from build123d import *

# Parameters (mm, degrees)
SKETCH1_W           = 57
SKETCH1_H           = 24.4
BOSS_EXTRUDE1_DEPTH = 1.2
SKETCH2_R           = 1.5
CUT_EXTRUDE1_DEPTH  = 2.2
SKETCH3_W           = 6
SKETCH3_H           = 8
BOSS_EXTRUDE2_DEPTH = 4
BOSS_EXTRUDE3_DEPTH = 4
SKETCH5_W           = 5
SKETCH5_H           = 8
BOSS_EXTRUDE4_DEPTH = 8.8
SKETCH6_W           = 3.7
SKETCH6_H           = 6.25
BOSS_EXTRUDE5_DEPTH = 4
SKETCH7_W           = 43.18
SKETCH7_H           = 2.54
BOSS_EXTRUDE6_DEPTH = 2.5
SKETCH8_W           = 0.65
SKETCH8_H           = 0.65
BOSS_EXTRUDE7_DEPTH = 5.9


with BuildPart() as part:
    # Sketch1 → Boss-Extrude1 (new body)
    with BuildSketch(Plane(origin=(0, 0, 0), x_dir=(1, 0, 0), z_dir=(0, 1, 0))):
        Rectangle(SKETCH1_W, SKETCH1_H)
    extrude(amount=BOSS_EXTRUDE1_DEPTH)

    # Sketch2 → Cut-Extrude1 (cut, through all)
    with BuildSketch(Plane(origin=(0, 1.2, 0), x_dir=(1, 0, 0), z_dir=(0, 1, 0))):
        with Locations((-26.035, -9.525)):
            Circle(SKETCH2_R)
        with Locations((26.035, -9.525)):
            Circle(SKETCH2_R)
        with Locations((26.035, 9.525)):
            Circle(SKETCH2_R)
        with Locations((-26.035, 9.525)):
            Circle(SKETCH2_R)
    extrude(amount=-CUT_EXTRUDE1_DEPTH, mode=Mode.SUBTRACT)

    # Sketch3 → Boss-Extrude2 (add)
    with BuildSketch(Plane(origin=(0, 1.2, 0), x_dir=(1, 0, 0), z_dir=(0, 1, 0))):
        with Locations((-25.5, 0)):
            Rectangle(SKETCH3_W, SKETCH3_H)
    extrude(amount=BOSS_EXTRUDE2_DEPTH)

    # Sketch4 → Boss-Extrude3 (add)
    with BuildSketch(Plane(origin=(0, 1.2, 0), x_dir=(1, 0, 0), z_dir=(0, 1, 0))):
        with BuildLine():
            Line((-16.25, -3.4), (-16.25, 3.4))
            ThreePointArc((-16.25, 3.4), (-14.5, 5.15), (-12.75, 3.4))
            Line((-12.75, 3.4), (-12.75, -3.4))
            ThreePointArc((-12.75, -3.4), (-14.5, -5.15), (-16.25, -3.4))
        make_face()
    extrude(amount=BOSS_EXTRUDE3_DEPTH)

    # Sketch5 → Boss-Extrude4 (add)
    with BuildSketch(Plane(origin=(0, 1.2, 0), x_dir=(1, 0, 0), z_dir=(0, 1, 0))):
        with Locations((13, 0)):
            Rectangle(SKETCH5_W, SKETCH5_H)
    extrude(amount=BOSS_EXTRUDE4_DEPTH)

    # Sketch6 → Boss-Extrude5 (add)
    with BuildSketch(Plane(origin=(0, 1.2, 0), x_dir=(1, 0, 0), z_dir=(0, 1, 0))):
        with Locations((19.05, 0)):
            Rectangle(SKETCH6_W, SKETCH6_H)
    extrude(amount=BOSS_EXTRUDE5_DEPTH)

    # Sketch7 → Boss-Extrude6 (add)
    with BuildSketch(Plane.XZ):
        with Locations((0, 8.89)):
            Rectangle(SKETCH7_W, SKETCH7_H)
        with Locations((0, -8.89)):
            Rectangle(SKETCH7_W, SKETCH7_H)
    extrude(amount=BOSS_EXTRUDE6_DEPTH)

    # Sketch8 → Boss-Extrude7 (add)
    with BuildSketch(Plane.XZ.offset(2.5)):
        with Locations((-17.78, 8.89)):
            Rectangle(SKETCH8_W, SKETCH8_H)
        with Locations((-20.32, 8.89)):
            Rectangle(SKETCH8_W, SKETCH8_H)
        with Locations((-15.24, 8.89)):
            Rectangle(SKETCH8_W, SKETCH8_H)
        with Locations((-12.7, 8.89)):
            Rectangle(SKETCH8_W, SKETCH8_H)
        with Locations((-10.16, 8.89)):
            Rectangle(SKETCH8_W, SKETCH8_H)
        with Locations((-7.62, 8.89)):
            Rectangle(SKETCH8_W, SKETCH8_H)
        with Locations((-5.08, 8.89)):
            Rectangle(SKETCH8_W, SKETCH8_H)
        with Locations((-2.54, 8.89)):
            Rectangle(SKETCH8_W, SKETCH8_H)
        with Locations((0, 8.89)):
            Rectangle(SKETCH8_W, SKETCH8_H)
        with Locations((2.54, 8.89)):
            Rectangle(SKETCH8_W, SKETCH8_H)
        with Locations((5.08, 8.89)):
            Rectangle(SKETCH8_W, SKETCH8_H)
        with Locations((7.62, 8.89)):
            Rectangle(SKETCH8_W, SKETCH8_H)
        with Locations((10.16, 8.89)):
            Rectangle(SKETCH8_W, SKETCH8_H)
        with Locations((12.7, 8.89)):
            Rectangle(SKETCH8_W, SKETCH8_H)
        with Locations((15.24, 8.89)):
            Rectangle(SKETCH8_W, SKETCH8_H)
        with Locations((17.78, 8.89)):
            Rectangle(SKETCH8_W, SKETCH8_H)
        with Locations((20.32, 8.89)):
            Rectangle(SKETCH8_W, SKETCH8_H)
        with Locations((20.32, -8.89)):
            Rectangle(SKETCH8_W, SKETCH8_H)
        with Locations((17.78, -8.89)):
            Rectangle(SKETCH8_W, SKETCH8_H)
        with Locations((15.24, -8.89)):
            Rectangle(SKETCH8_W, SKETCH8_H)
        with Locations((12.7, -8.89)):
            Rectangle(SKETCH8_W, SKETCH8_H)
        with Locations((10.16, -8.89)):
            Rectangle(SKETCH8_W, SKETCH8_H)
        with Locations((7.62, -8.89)):
            Rectangle(SKETCH8_W, SKETCH8_H)
        with Locations((5.08, -8.89)):
            Rectangle(SKETCH8_W, SKETCH8_H)
        with Locations((2.54, -8.89)):
            Rectangle(SKETCH8_W, SKETCH8_H)
        with Locations((0, -8.89)):
            Rectangle(SKETCH8_W, SKETCH8_H)
        with Locations((-2.54, -8.89)):
            Rectangle(SKETCH8_W, SKETCH8_H)
        with Locations((-5.08, -8.89)):
            Rectangle(SKETCH8_W, SKETCH8_H)
        with Locations((-7.62, -8.89)):
            Rectangle(SKETCH8_W, SKETCH8_H)
        with Locations((-10.16, -8.89)):
            Rectangle(SKETCH8_W, SKETCH8_H)
        with Locations((-12.7, -8.89)):
            Rectangle(SKETCH8_W, SKETCH8_H)
        with Locations((-15.24, -8.89)):
            Rectangle(SKETCH8_W, SKETCH8_H)
        with Locations((-17.78, -8.89)):
            Rectangle(SKETCH8_W, SKETCH8_H)
        with Locations((-20.32, -8.89)):
            Rectangle(SKETCH8_W, SKETCH8_H)
    extrude(amount=BOSS_EXTRUDE7_DEPTH)


solid = part.part
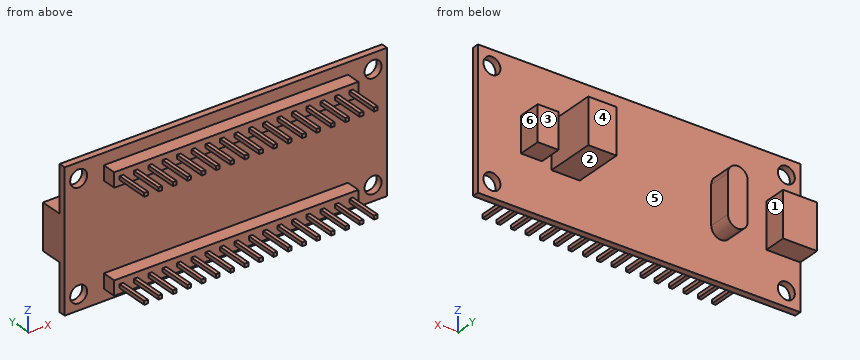
Work out the finished part from the listing and answer in its coordinate system (mm). Face numbers are marked on the shaded views. A direction names the side the tool comes from. Give positions to 0.01 mm unless a question says otherwise; leave off trailing zeros. Loops run counter-clockwise (first coordinate to the right, second up) from the corner with the lowest first, then second, coordinate; pieces in that order, holes last. Notation, with made-up numbers: (79, 75.5) - (87, 75.5) arc R12 cw to (87, 95.5) - close; hole circle Ø10 at (49, 53.5). An arc over 180 degrees is marked (long way). Answer in a Markdown table with one row per item. Add a question column.
Q1. A tool of negligible diameter and unlimited length cuts with its end or side. For the marked faces 1, 2 and 3, from which of +Z, -Z, +X, -X, +Y, -Y can it reach the whole face along a straight path? Write none if from no direction.
Q2. The part is cut by section C-C (y = 7). Determine the outline of the cut face in (x, z), and give its area (3 significant figures).
Q3. Each of these flat-tipped pins is pushed along its axis until it touches: P1, Ø0.7, axis at x = 0, y = -6, coming from the +Z side (3 decimals); P2, Ø3, axis at y = 2, z = -3.5, coming from the +X side; P3, Ø0.7, axis at y = -6.5, z = -9, coming from the -X side (3 decimals); P4, Ø5, axis at x = 0.5, y = -4.5, coming from the -Z side. Where does it stop, or does it pass through?
Q4. The part is cut by section A-A (x = -1). Determine the outline of the cut face in (y, z), and give its area (3 significant figures).
Q5. The part is cut by section B-B (z = -1). Determine the outline of the cut face in (x, y).
Q6. Consider line 1 along Z through (x, y) = (-7, -0.5); line 2 along Y through (x, z) = (-8.5, 2.75); line 3 along Y through (x, z) = (14.5, 0). Determine where each line is inside the solid, lowest interval first.
Q7. Determine the mould class of the marked faces 4, 5 and 6 for opening direction X: released by +X, released by -X, zero draft, split by the parting line, or undercut.
Q8. The part is cut by section D-D (x = 22.5). Determine the outline of the cut face in (y, z), and give its area (3 significant figures).
Solution:
| question | item | result |
|---|---|---|
| 1 | face 1 | +Z, -Z, +Y |
| 1 | face 2 | -Z, +X, +Y |
| 1 | face 3 | +Z, -Z, +X, +Y |
| 2 | outline | (10.5, -4) - (15.5, -4) - (15.5, 4) - (10.5, 4) - close |
| 2 | area | 40.0 mm² |
| 3 | P1 | stops at z = 9.215 |
| 3 | P2 | stops at x = 28.5 |
| 3 | P3 | stops at x = -20.645 |
| 3 | P4 | stops at z = -10.16 |
| 4 | outline | (-2.5, -10.16) - (0, -10.16) - (0, -12.2) - (1.2, -12.2) - (1.2, 12.2) - (0, 12.2) - (0, 10.16) - (-2.5, 10.16) - (-2.5, 7.62) - (0, 7.62) - (0, -7.62) - (-2.5, -7.62) - close |
| 4 | area | 42.0 mm² |
| 5 | outline | (-28.5, 0) - (28.5, 0) - (28.5, 1.2) - (20.9, 1.2) - (20.9, 5.2) - (17.2, 5.2) - (17.2, 1.2) - (15.5, 1.2) - (15.5, 10) - (10.5, 10) - (10.5, 1.2) - (-12.75, 1.2) - (-12.75, 5.2) - (-16.25, 5.2) - (-16.25, 1.2) - (-22.5, 1.2) - (-22.5, 5.2) - (-28.5, 5.2) - close |
| 6 | line 1 | z = -10.16 to -7.62, 7.62 to 10.16 |
| 6 | line 2 | y = 0 to 1.2 |
| 6 | line 3 | y = 0 to 10 |
| 7 | face 4 | zero draft |
| 7 | face 5 | undercut |
| 7 | face 6 | released by +X |
| 8 | outline | (0, -12.2) - (1.2, -12.2) - (1.2, 12.2) - (0, 12.2) - close |
| 8 | area | 29.3 mm² |
